The model under review builds one solid part; all positions refer to its coordinate system, in mm. Face numbers are marked on the shaded views. A direction names the side the tool comes from. Coordinates: 2 decimals unless noted, no trailing zeros. Loops run counter-clockwise (first coordinate to the right, second up) from the corner with the lowest first, then second, coordinate; pieces in that order, holes last. Notation, with made-up numbers: M -36.5,0.5 L -30.5,0.5 A21 ccw -30.5,32.5 Z; hole C -12,55 d9. An arc over 180 degrees is marked long. Use CSV: the item, a comma, the result in double quotes. Start each with the question number.
1. Draft analysis for pull direction Z (two halves, no side actions). For the marked faces 5, 6 and 7, state which applies: +Z half, -Z half, draft (parallel to the pull), parting line (faces both ways), or undercut.
2. Add section B-B, the plane z = -15. State how many separate pieces and enclosed holes the cut face has, then the cut area to 3 significant figures.
3. For L1, parallel to Z at x = 28.5, y = 14.5; L2, parallel to Z at x = 18, y = 20; L3, parallel to Y at x = 27.25, z = -15 (3 decimals), list the stretches that pass through material, from the lowest coordinate up.
4. Clearance check with flat-ended pins moving along their axes: P1, Ø5, axis at y = 127.5, z = -5.5, coming from the -X side; P2, Ø9, axis at x = -21, z = -20, coming from the -Y side; P3, Ø11, axis at y = 6.56, z = -15, coming from the +X side; P4, Ø2.5, axis at x = 15, z = -27, coming from the -Y side. State where each tip first meets the part, or that it passes through.
5. Add section A-A, the plane y = 15.06. Write out the cut boundary in (x, z) (3 decimals), then the cut area to 4 significant figures.
6. Add section D-D, the plane y = 75. Write out the cut boundary in (x, z).
7. Tool access review of the marked faces 1, 2, 3 and 4: name each direction out of +Z, -Z, +X, -X, +Y, -Y from which nothing blocks a thin tool from reaching the whole face with its end or side.
8. Add section C-C, the plane z = -26.5. Write out the cut boundary in (x, y).
Autodesk Inventor part; units mm, degrees
ref_plane "YZ Plane" through (0, 0, 0) normal (1, 0, 0) x (0, 1, 0)
ref_plane "XZ Plane" through (0, 0, 0) normal (0, 1, 0) x (-1, 0, 0)
ref_plane "XY Plane" through (0, 0, 0) normal (0, 0, 1) x (1, 0, 0)
sketch "Sketch1" plane through (0, 0, 0) normal (0, 0, 1) x (1, 0, 0)
  line L0 (0, 0) -> (25, 0)
  line L1 (25, 0) -> (25, 40)
  line L2 (25, 40) -> (0, 40)
  line L3 (0, 40) -> (0, 0)
  dimension "d1" = 25
  dimension "d2" = 40
  dimension "d3" = 25
extrude "Extrusion1" add sketch "Sketch1" against normal blind 30
sketch "Sketch2" plane through (25, 0, 0) normal (1, 0, 0) x (0, 0, -1)
  line L0 (0, 0) -> (30, 0)
  circle A0 centre (15, 6.56) radius 2.46
extrude "Extrusion2" cut sketch "Sketch2" against normal blind 30
sketch "Sketch3" plane through (0, 0, 0) normal (-1, 0, 0) x (0, 0, 1)
  line L0 (0, 0) -> (-30, 0)
  line L1 (-25.05, 0) -> (-4.95, 0)
  line L2 (-4.95, 0) -> (-4.95, 33.12)
  line L3 (-4.95, 33.12) -> (-25.05, 33.12)
  line L4 (-25.05, 33.12) -> (-25.05, 0)
  dimension "d11" = 20.1
extrude "Extrusion3" cut sketch "Sketch3" against normal blind 20
sketch "Sketch4" plane through (0, 0, 0) normal (0, -1, 0) x (1, 0, 0)
  line L0 (20, -4.95) -> (20, -25.05)
  line L1 (20, -15) -> (25, -15)
  line L2 (25, 0) -> (25, -30)
  line L3 (20, -8.025) -> (25, -8.025)
  line L4 (25, -8.025) -> (25, -21.975)
  line L5 (25, -21.975) -> (20, -21.975)
  line L6 (20, -21.975) -> (20, -8.025)
  line L7 (20, -8.025) -> (25, -21.975) construction
  line L8 (25, -8.025) -> (20, -21.975) construction
  line L9 (25, -12.54) -> (25, -17.46)
  point P0 (0, 0)
  point P1 (22.5, -15)
  dimension "d14" = 13.95
extrude "Extrusion4" add sketch "Sketch4" along normal blind 15
sketch "Sketch5" plane through (20, 0, 0) normal (-1, 0, 0) x (0, 0, 1)
  circle A0 centre (-15, 6.56) radius 2.46
  circle A1 centre (-15, 6.56) radius 4.7025
  circle A2 centre (-15, 6.56) radius 2.46
  circle A3 centre (-15, 6.56) radius 2.46
  point P0 (0, 0)
  dimension "d17" = 9.405
extrude "Extrusion5" cut sketch "Sketch5" against normal blind 2.1
sketch "Sketch6" plane through (25, 0, 0) normal (1, 0, 0) x (0, 0, -1)
  circle A0 centre (15, 6.56) radius 4.7025
  line L0 (15, 6.56) -> (15, 23.56)
  circle A1 centre (15, 23.56) radius 2.46
  point P0 (0, 0)
  dimension "d20" = 17
  dimension "d21" = 4.92
extrude "Extrusion6" cut sketch "Sketch6" against normal blind 10 contours A1
sketch "Sketch7" plane through (20, 0, 0) normal (-1, 0, 0) x (0, 0, 1)
  circle A0 centre (-15, 23.56) radius 2.46
  circle A1 centre (-15, 23.56) radius 4.7025
  point P0 (0, 0)
  dimension "d24" = 9.405
extrude "Extrusion7" cut sketch "Sketch7" against normal blind 2.1
sketch "Sketch9" plane through (25, 0, 0) normal (1, 0, 0) x (0, 0, -1)
  circle A0 centre (15, 6.56) radius 2.46
  circle A1 centre (15, 6.56) radius 2.46
  circle A2 centre (15, 23.56) radius 2.46
  circle A3 centre (15, 23.56) radius 2.46
  line L0 (30, 40) -> (30, 0)
  line L1 (30, 0) -> (30, 40)
  line L2 (30, 40) -> (0, 40)
  line L3 (0, 40) -> (0, 0)
  line L4 (0, 0) -> (8.025, 0)
  line L5 (21.975, 0) -> (21.975, -15)
  line L6 (21.975, -15) -> (8.025, -15)
  line L7 (8.025, -15) -> (8.025, 0)
  line L8 (0, 0) -> (8.025, 0)
  line L9 (21.975, 0) -> (30, 0)
extrude "Extrusion8" add sketch "Sketch9" along normal blind 5
sketch "Sketch10" plane through (0, 40, 0) normal (0, 1, 0) x (1, 0, 0)
  line L0 (0, 30) -> (30, 30)
  line L1 (30, 0) -> (0, 0)
  line L2 (0, 30) -> (30, 30)
  line L3 (30, 30) -> (30, 0)
  line L4 (30, 0) -> (0, 0)
  line L5 (0, 0) -> (0, 30)
extrude "Extrusion9" add sketch "Sketch10" along normal blind 30
sketch "Sketch12" plane through (30, 0, 0) normal (1, 0, 0) x (0, 0, -1)
  circle A0 centre (15, 6.56) radius 2.46
  line L0 (15, 6.56) -> (15, 15.06)
  circle A1 centre (15, 15.06) radius 2.525
  point P0 (0, 0)
  dimension "d31" = 8.5
  dimension "d33" = 5.05
extrude "Extrusion10" cut sketch "Sketch12" against normal blind 30 contours A1
sketch "Sketch14" plane through (0, 0, 0) normal (0, 0, 1) x (1, 0, 0)
  line L0 (30, 70) -> (0, 70)
  line L1 (0, 70) -> (0, 85)
  line L2 (-15, 100) -> (-23, 100)
  line L3 (30, 0) -> (30, 70)
  line L4 (30, 122.5) -> (30, 70)
  arc A0 (0, 85) -> (-15, 100) centre (-15, 85) ccw
  line L5 (30, 105) -> (30, 100)
  line L6 (-23, 153) -> (15, 153)
  line L7 (-18, 150.5) -> (-23, 153)
  line L8 (-18, 102.5) -> (-23, 100)
  line L9 (-18, 102.5) -> (-13, 126.5)
  line L10 (-13, 126.5) -> (-18, 150.5)
  line L11 (30, 126.5) -> (15, 153)
  line L12 (30, 122.5) -> (30, 126.5)
  point P0 (0, 0)
  point P1 (0, 100)
  dimension "d47" = 30
  dimension "d54" = 15
extrude "Extrusion12" add sketch "Sketch14" against normal blind 30
sketch "Sketch15" plane through (0, 0, -25.05) normal (-1, 0, 0) x (0, 0, 1)
  line L0 (0, 33.12) -> (20.1, 33.12)
  line L1 (20.1, 33.12) -> (20.1, 0)
  line L2 (0, 33.12) -> (20.1, 33.12)
  line L3 (20.1, 33.12) -> (20.1, 31.1)
  line L4 (20.1, 31.1) -> (0, 31.1)
  line L5 (0, 31.1) -> (0, 33.12)
  point P0 (25.05, 0)
  dimension "d57" = 2.02
extrude "Extrusion13" add sketch "Sketch15" against normal blind 20
properties part number "rec_a_48mm_x_30mm"
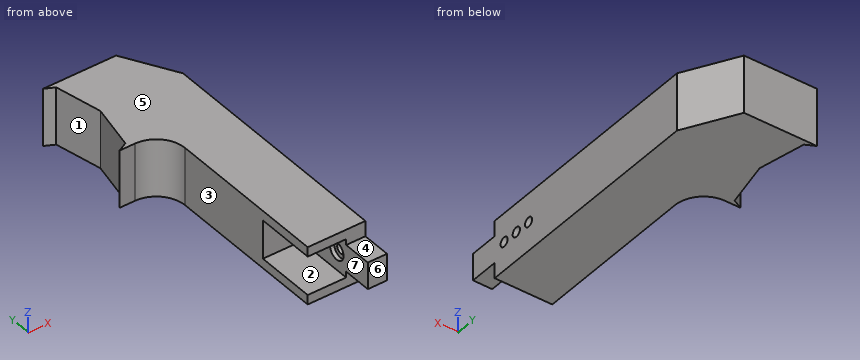
Computed:
1,face 5,"+Z half"
1,face 6,"draft"
1,face 7,"undercut"
2,separate pieces,"4"
2,enclosed holes,"0"
2,area,"4,650 mm^2"
3,L1,"z = -30 to -17.46, -12.54 to 0"
3,L2,"z = -30 to -25.05, -4.95 to 0"
3,L3,"y = -15 to 4.1, 9.02 to 12.535, 17.585 to 21.1, 26.02 to 131.358"
4,P1,"stops at x = -13.73"
4,P2,"stops at y = 100"
4,P3,"stops at x = 30"
4,P4,"stops at y = 0"
5,outline,"M 0,-30 L 30,-30 L 30,-17.525 L 20,-17.525 L 20,-25.05 L 0,-25.05 Z; M 0,-4.95 L 20,-4.95 L 20,-12.475 L 30,-12.475 L 30,0 L 0,0 Z"
5,area,"447.5 mm^2"
6,outline,"M 0,-30 L 30,-30 L 30,0 L 0,0 Z"
7,face 1,"+Z, -Z, -X"
7,face 2,"-X, -Y"
7,face 3,"+Z, -Z, -X, -Y"
7,face 4,"+Z, +X, -X, -Y"
8,outline,"M -23,100 L -15,100 A15 cw 0,85 L 0,0 L 30,0 L 30,126.5 L 15,153 L -23,153 L -18,150.5 L -13,126.5 L -18,102.5 Z"
